Read the model definition and answer for the solid it produces. Units are mm, in the model's axes. A direction names the side the tool comes from. Coordinates: 2 decimals unless noted, no trailing zeros. Write each loop counter-clockwise with the first axis right and the second up, starting at its lowest first coordinate (ties: lowest second). Pieces come first, ordered by that corner, then holes. Notation, with made-up numbers: M -6.75,12.25 L 3.25,12.25 A20 cw 3.25,40.25 Z; hole C -25.75,82 d1. An arc over 180 degrees is marked long. Write item = value, one per line.
from build123d import *

# Parameters (mm, degrees)
F0_W     = 56.5631985664
F0_H     = 35.8275994658
F1_DEPTH = 330
F2_DEPTH = 300
F3_DEPTH = 300
F4_R     = 7
F5_T     = -1


with BuildPart() as f1:
    # F0 (on Top) → F1 (new body)
    with BuildSketch(Plane.XY):
        with Locations((28.2815992832, 17.9137997329)):
            Rectangle(F0_W, F0_H)
    extrude(amount=F1_DEPTH)

    # F2 (add): a face of the model
    f2_faces = [f1.faces().sort_by_distance(p)[0] for p in [
        (0, 17.9137997329, 165),
    ]]
    extrude(f2_faces, amount=-F2_DEPTH)

    # F3 (add): a face of the model
    f3_faces = [f1.faces().sort_by_distance(p)[0] for p in [
        (150, 0, 165),
    ]]
    extrude(f3_faces, amount=-F3_DEPTH)

    # F4
    f4_edges = [f1.edges().sort_by_distance(p)[0] for p in [
        (0, 0, 165),
        (300, 0, 165),
    ]]
    fillet(f4_edges, radius=F4_R)

    # F5
    f5_openings = [f1.faces().sort_by_distance(p)[0] for p in [
        (150, 150.034694, 330),
        (150, 300, 165),
        (150, 150.034694, 0),
    ]]
    offset(amount=F5_T, openings=f5_openings)


solid = f1.part
Item 1: A flat-ended cylindrical pin translates along its axis: pin 1 (4 mm diameter, centred on x = 240.5, z = 210, fed in from +Y). Find the tip coordinate at first contact, or state that the pin passes through.
Worked answers:
pin_1 = 1
Item 2: Consider line 1 along X through (y, z) = (211.5, 268); line 2 along Y through (x, z) = (192.5, 224.5). Determine where each line is inside the solid, lowest interval first. Write a range as from..to.
Worked answers:
line_1 = 0..1, 299..300
line_2 = 0..1
Item 3: Find section A-A (y = 163). Determine the outline of the cut face in (x, z).
Worked answers:
outline = M 0,0 L 1,0 L 1,330 L 0,330 Z; M 299,0 L 300,0 L 300,330 L 299,330 Z
Item 4: For a pull along X with two mould halves and no side action, classify faces 1 (the face through (1, 151, 163)), 2 (the face through (0, 151, 163)), 3 (the face through (148, 0, 163)) as released by +X, released by -X, zero draft, split by the parting line, or undercut.
Worked answers:
face_1 = undercut
face_2 = released by -X
face_3 = zero draft
Item 5: Find section B-B (z = 209). Determine the outline of the cut face in (x, y).
Worked answers:
outline = M 0,7 A7 ccw 7,0 L 293,0 A7 ccw 300,7 L 300,300 L 299,300 L 299,7 A6 cw 293,1 L 7,1 A6 cw 1,7 L 1,300 L 0,300 Z
Item 6: Which of the six approach directions +Z, -Z, +X, -X, +Y, -Y give full straight-line access (tool end or side, diameter ignored) to faces 4 (the face through (300, 151, 163)), 5 (the face through (299, 151, 163))?
Worked answers:
face_4 = +Z, -Z, +X, +Y, -Y
face_5 = +Z, -Z, +Y
Item 7: Find section C-C (x = 87). Determine the outline of the cut face in (y, z), and give its area (3 significant figures).
Worked answers:
outline = M 0,0 L 1,0 L 1,330 L 0,330 Z
area = 330 mm²
